```python
from build123d import *

# Parameters (mm, degrees)
CYLINDER002_R               = 34.5
CYLINDER002_DEPTH           = 20
COMPOUND_PLACEMENT_ANGLE    = 45
CYLINDER003_R               = 34.5
CYLINDER003_DEPTH           = 20
COMPOUND001_PLACEMENT_ANGLE = 90
CYLINDER004_R               = 34.5
CYLINDER004_DEPTH           = 20
COMPOUND002_PLACEMENT_ANGLE = 135
CYLINDER005_R               = 34.5
CYLINDER005_DEPTH           = 20
COMPOUND003_PLACEMENT_ANGLE = 180
CYLINDER006_R               = 34.5
CYLINDER006_DEPTH           = 20
COMPOUND004_PLACEMENT_ANGLE = 225
CYLINDER007_R               = 34.5
CYLINDER007_DEPTH           = 20
COMPOUND005_PLACEMENT_ANGLE = 270
CYLINDER008_R               = 34.5
CYLINDER008_DEPTH           = 20
COMPOUND006_PLACEMENT_ANGLE = 315
CYLINDER_R                  = 34.5
CYLINDER_DEPTH              = 20
EXTRUDE001_DEPTH            = 80
EXTRUDE_DEPTH               = 80


with BuildPart() as compound:
    # Cylinder002 → Cylinder002 (new body)
    with BuildSketch(Plane.XZ.offset(-179.75)):
        Circle(CYLINDER002_R)
    extrude(amount=CYLINDER002_DEPTH)


with BuildPart() as compound_1:
    # Compound placement: moved
    add(compound.part.rotate(Axis((0, 0, 0), (0, 0, 1)), COMPOUND_PLACEMENT_ANGLE))


with BuildPart() as compound001:
    # Cylinder003 → Cylinder003 (new body)
    with BuildSketch(Plane.XZ.offset(-179.75)):
        Circle(CYLINDER003_R)
    extrude(amount=CYLINDER003_DEPTH)


with BuildPart() as compound001_1:
    # Compound001 placement: moved
    add(compound001.part.rotate(Axis((0, 0, 0), (0, 0, 1)), COMPOUND001_PLACEMENT_ANGLE))


with BuildPart() as compound002:
    # Cylinder004 → Cylinder004 (new body)
    with BuildSketch(Plane.XZ.offset(-179.75)):
        Circle(CYLINDER004_R)
    extrude(amount=CYLINDER004_DEPTH)


with BuildPart() as compound002_1:
    # Compound002 placement: moved
    add(compound002.part.rotate(Axis((0, 0, 0), (0, 0, 1)), COMPOUND002_PLACEMENT_ANGLE))


with BuildPart() as compound003:
    # Cylinder005 → Cylinder005 (new body)
    with BuildSketch(Plane.XZ.offset(-179.75)):
        Circle(CYLINDER005_R)
    extrude(amount=CYLINDER005_DEPTH)


with BuildPart() as compound003_1:
    # Compound003 placement: moved
    add(compound003.part.rotate(Axis((0, 0, 0), (0, 0, 1)), COMPOUND003_PLACEMENT_ANGLE))


with BuildPart() as compound004:
    # Cylinder006 → Cylinder006 (new body)
    with BuildSketch(Plane.XZ.offset(-179.75)):
        Circle(CYLINDER006_R)
    extrude(amount=CYLINDER006_DEPTH)


with BuildPart() as compound004_1:
    # Compound004 placement: moved
    add(compound004.part.rotate(Axis((0, 0, 0), (0, 0, 1)), COMPOUND004_PLACEMENT_ANGLE))


with BuildPart() as compound005:
    # Cylinder007 → Cylinder007 (new body)
    with BuildSketch(Plane.XZ.offset(-179.75)):
        Circle(CYLINDER007_R)
    extrude(amount=CYLINDER007_DEPTH)


with BuildPart() as compound005_1:
    # Compound005 placement: moved
    add(compound005.part.rotate(Axis((0, 0, 0), (0, 0, 1)), COMPOUND005_PLACEMENT_ANGLE))


with BuildPart() as compound006:
    # Cylinder008 → Cylinder008 (new body)
    with BuildSketch(Plane.XZ.offset(-179.75)):
        Circle(CYLINDER008_R)
    extrude(amount=CYLINDER008_DEPTH)


with BuildPart() as compound006_1:
    # Compound006 placement: moved
    add(compound006.part.rotate(Axis((0, 0, 0), (0, 0, 1)), COMPOUND006_PLACEMENT_ANGLE))


with BuildPart() as compound007:
    # Cylinder → Cylinder (new body)
    with BuildSketch(Plane.XZ.offset(-179.75)):
        Circle(CYLINDER_R)
    extrude(amount=CYLINDER_DEPTH)

    # Compound007: union Compound, Compound001, Compound002, Compound003, Compound004, Compound005, Compound006
    add(compound_1.part)
    add(compound001_1.part)
    add(compound002_1.part)
    add(compound003_1.part)
    add(compound004_1.part)
    add(compound005_1.part)
    add(compound006_1.part)


with BuildPart() as extrude001:
    # Wire001 → Extrude001 (new body)
    with BuildSketch(Plane.XY.offset(-40)):
        Polygon((66.59, 160.76), (160.76, 66.59), (160.76, -66.59), (66.59, -160.76), (-66.59, -160.76), (-160.76, -66.59), (-160.76, 66.59), (-66.59, 160.76), align=None)
    extrude(amount=EXTRUDE001_DEPTH)


with BuildPart() as cut001:
    # Wire → Extrude (new body)
    with BuildSketch(Plane.XY.offset(-40)):
        Polygon((74.24, 179.24), (179.24, 74.24), (179.24, -74.24), (74.24, -179.24), (-74.24, -179.24), (-179.24, -74.24), (-179.24, 74.24), (-74.24, 179.24), align=None)
    extrude(amount=EXTRUDE_DEPTH)

    # Cut: cut Extrude001
    add(extrude001.part, mode=Mode.SUBTRACT)

    # Cut001: cut Compound007
    add(compound007.part, mode=Mode.SUBTRACT)


solid = cut001.part
```
Here's how the part is built. I have some questions about the finished solid (model axes, mm). A direction names the side the tool comes from. Coordinates: 2 decimals unless noted, no trailing zeros. Order: outer loops, then holes, each group sorted by start corner. A loop starts at its lowest first (then second) coordinate and runs counter-clockwise, first axis right, second up. Notation, with made-up numbers: M 7,59 L 18,59 A15 cw 18,68 Z; hole C -23,4 d2. An arc over 180 degrees is marked long. Answer as a JSON object with one key per item and string values. Group by question number.
(1) Suppose I cut it at C-C, the plane x = -43. Please give me the cut outline in (y, z), then the cut area to 3 significant figures.
(2) Which directions (+Z, -Z, +X, -X, +Y, -Y) give clear straight access to the entire face, cutting with the end or side of a thin tool? Please do faces 1 (the face through (92.09, 135.26, 17.22)), 2 (the face through (102.32, 138.28, 23.32)).
(3) For pin 1 (24 mm diameter, centred on x = 21, z = 8.5, fed in from +Y); pin 2 (2 mm diameter, centred on x = -78.5, z = 28.5, fed in from +Y); pin 3 (4 mm diameter, centred on x = 91.5, z = -5.5, fed in from +Y), each with a flat end and sliding along its axis, tell me the tip position at first contact or that it passes through.
(4) Suppose I cut it at D-D, the plane z = 11.5. State how many separate pieces and enclosed holes the cut face has, then the cut area to 3 significant figures.
(5) Suppose I cut it at A-A, the plane y = 0. Please give me the cut outline in (x, z), then the cut area to 3 significant figures.
(6) I need wall thicknesses on probe 1 along X at (y, z) = (36, 10.5); probe 2 along Z at (x, y) = (0, -174.5). Which ranges of each line are inside material? Lowest first, please.
(7) If we mould it in two halves opening along Z, with no side actions, what happens to faces 3 (the face through (94, 134, 40)), 4 (the face through (-150.81, 102.67, 8.33)), 5 (the face through (-143.57, -97.03, 10.36)), 6 (the face through (94, 134, -40))? For each: released by +Z, released by -Z, zero draft, split by the parting line, or undercut.
Values found:
{
 "1": {"outline": "M -179.24,-40 L -160.76,-40 L -160.76,40 L -179.24,40 Z; M 160.76,-40 L 179.24,-40 L 179.24,40 L 160.76,40 Z", "area": "2,960 mm^2"},
 "2": {"face 1": "+Z, -Z", "face 2": "none"},
 "3": {"pin 1": "stops at y = 179.24", "pin 2": "stops at y = 175.98", "pin 3": "stops at y = 163.98"},
 "4": {"separate pieces": "8", "enclosed holes": "0", "area": "11,200 mm^2"},
 "5": {"outline": "M -179.24,-40 L -160.76,-40 L -160.76,-34.5 L -179.24,-34.5 Z; M -179.24,34.5 L -160.76,34.5 L -160.76,40 L -179.24,40 Z; M 160.76,-40 L 179.24,-40 L 179.24,-34.5 L 160.76,-34.5 Z; M 160.76,34.5 L 179.24,34.5 L 179.24,40 L 160.76,40 Z", "area": "407 mm^2"},
 "6": {"probe 1": "x = -179.24 to -160.76, 160.76 to 179.24", "probe 2": "z = -40 to -34.5, 34.5 to 40"},
 "7": {"face 3": "released by +Z", "face 4": "zero draft", "face 5": "undercut", "face 6": "released by -Z"}
}
